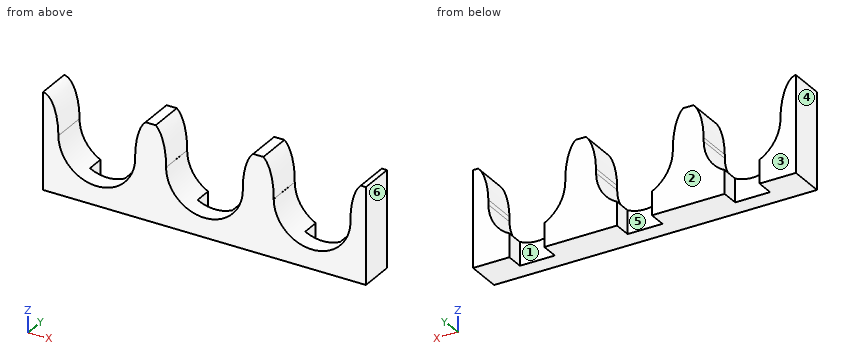
from build123d import *

# Parameters (mm, degrees)
SKETCH1_W           = 469.9
SKETCH1_H           = 139.7
BOSS_EXTRUDE1_DEPTH = 50.8
SKETCH2_R           = 55.88
CUT_EXTRUDE3_DEPTH  = 405.871109401
CUT_EXTRUDE5_DEPTH  = 405.871109401
SKETCH5_W           = 50.8
SKETCH5_H           = 25.4
CUT_EXTRUDE6_DEPTH  = 419.118003235


with BuildPart() as part:
    # Sketch1 → Boss-Extrude1 (new body)
    with BuildSketch(Plane(origin=(0, 0, 0), x_dir=(1, 0, 0), z_dir=(0, 1, 0))):
        with Locations((155.851656231, -22.96185654)):
            Rectangle(SKETCH1_W, SKETCH1_H)
    extrude(amount=BOSS_EXTRUDE1_DEPTH)

    # Sketch2 → Cut-Extrude3 (cut, through all)
    with BuildSketch(Plane(origin=(0, 50.8, 0), x_dir=(1, 0, 0), z_dir=(0, 1, 0))):
        with BuildLine():
            Line((55.098238231, -92.81185654), (55.098238231, -36.93185654))
            ThreePointArc((55.098238231, -36.93185654), (38.731365092, -76.444983544), (-0.781761972, -92.81185654))
            Line((-0.781761972, -92.81185654), (55.098238231, -92.81185654))
        make_face()
        with BuildLine():
            ThreePointArc((-0.781761972, -92.81185654), (-40.294888773, -76.4449834), (-56.661761769, -36.93185654))
            Line((-56.661761769, -36.93185654), (-56.661761769, -92.81185654))
            Line((-56.661761769, -92.81185654), (-0.781761972, -92.81185654))
        make_face()
        with BuildLine():
            Line((99.971656231, -36.93185654), (99.971656231, -92.81185654))
            Line((99.971656231, -92.81185654), (155.851656231, -92.81185654))
            ThreePointArc((155.851656231, -92.81185654), (116.338529299, -76.444983472), (99.971656231, -36.93185654))
        make_face()
        with BuildLine():
            ThreePointArc((211.731656231, -36.93185654), (195.364783164, -76.444983472), (155.851656231, -92.81185654))
            Line((155.851656231, -92.81185654), (211.731656231, -92.81185654))
            Line((211.731656231, -92.81185654), (211.731656231, -36.93185654))
        make_face()
        with BuildLine():
            Line((256.605074231, -36.93185654), (256.605074231, -92.81185654))
            Line((256.605074231, -92.81185654), (312.485074664, -92.81185654))
            ThreePointArc((312.485074664, -92.81185654), (272.971947451, -76.444983625), (256.605074231, -36.93185654))
        make_face()
        with BuildLine():
            ThreePointArc((368.365074231, -36.93185654), (351.998201317, -76.444983319), (312.485074664, -92.81185654))
            Line((312.485074664, -92.81185654), (368.365074231, -92.81185654))
            Line((368.365074231, -92.81185654), (368.365074231, -36.93185654))
        make_face()
        with Locations((312.485074231, -36.93185654)):
            Circle(SKETCH2_R)
        with Locations((155.851656231, -36.93185654)):
            Circle(SKETCH2_R)
        with Locations((-0.781761769, -36.93185654)):
            Circle(SKETCH2_R)
    extrude(amount=-CUT_EXTRUDE3_DEPTH, mode=Mode.SUBTRACT)

    # Sketch3 → Cut-Extrude5 (cut, through all)
    with BuildSketch(Plane(origin=(0, 50.8, 0), x_dir=(1, 0, 0), z_dir=(0, 1, 0))):
        with BuildLine():
            Line((-56.661761769, -92.81185654), (-56.661761769, -36.93185654))
            add(Edge.make_bspline(
                [(-79.098343769, -92.81185654), (-56.661761769, -92.81185654), (-56.661761769, -36.93185654)],
                knots=[0, 0, 0, 1.570796327, 1.570796327, 1.570796327], degree=2, weights=[1, 0.707106781, 1]))
            Line((-79.098343769, -92.81185654), (-56.661761769, -92.81185654))
        make_face()
        with BuildLine():
            add(Edge.make_bspline(
                [(55.098238231, -42.266592873), (55.687318095, -80.198521665), (70.062894281, -92.81185654)],
                knots=[4.75104815, 4.75104815, 4.75104815, 5.944468502, 5.944468502, 5.944468502], degree=2, weights=[1, 0.82718872, 1]))
            Line((55.098238231, -42.266592873), (55.098238231, -92.81185654))
            Line((55.098238231, -92.81185654), (70.062894281, -92.81185654))
        make_face()
        with BuildLine():
            Line((99.971656231, -36.93185654), (99.918392881, -36.93185654))
            add(Edge.make_bspline(
                [(84.973218182, -92.81185654), (100.8764169, -78.858163942), (99.918392881, -36.93185654)],
                knots=[0.338716805, 0.338716805, 0.338716805, 1.627645124, 1.627645124, 1.627645124], degree=2, weights=[1, 0.799421799, 1]))
            Line((84.973218182, -92.81185654), (99.971656231, -92.81185654))
            Line((99.971656231, -92.81185654), (99.971656231, -36.93185654))
        make_face()
        with BuildLine():
            add(Edge.make_bspline(
                [(211.731656231, -43.172150916), (212.553221033, -80.41743909), (226.679294281, -92.81185654)],
                knots=[4.767271474, 4.767271474, 4.767271474, 5.944468502, 5.944468502, 5.944468502], degree=2, weights=[1, 0.831719595, 1]))
            Line((211.731656231, -43.172150916), (211.731656231, -92.81185654))
            Line((211.731656231, -92.81185654), (226.679294281, -92.81185654))
        make_face()
        with BuildLine():
            Line((256.605074231, -36.93185654), (256.534792881, -36.93185654))
            add(Edge.make_bspline(
                [(241.589618182, -92.81185654), (257.4928169, -78.858163942), (256.534792881, -36.93185654)],
                knots=[0.338716805, 0.338716805, 0.338716805, 1.627645124, 1.627645124, 1.627645124], degree=2, weights=[1, 0.799421799, 1]))
            Line((241.589618182, -92.81185654), (256.605074231, -92.81185654))
            Line((256.605074231, -92.81185654), (256.605074231, -36.93185654))
        make_face()
        with BuildLine():
            add(Edge.make_bspline(
                [(368.365074231, -43.865048297), (369.358856755, -80.583477202), (383.295694281, -92.81185654)],
                knots=[4.779694469, 4.779694469, 4.779694469, 5.944468502, 5.944468502, 5.944468502], degree=2, weights=[1, 0.835152126, 1]))
            Line((368.365074231, -43.865048297), (368.365074231, -92.81185654))
            Line((368.365074231, -92.81185654), (383.295694281, -92.81185654))
        make_face()
    extrude(amount=-CUT_EXTRUDE5_DEPTH, mode=Mode.SUBTRACT)

    # Sketch5 → Cut-Extrude6 (cut, through all)
    with BuildSketch(Plane(origin=(0, 0, -46.88814346), x_dir=(-1, 0, 0), z_dir=(0, 0, -1))):
        with Locations((-312.485836231, 38.1)):
            Rectangle(SKETCH5_W, SKETCH5_H)
        with Locations((-155.851656231, 38.1)):
            Rectangle(SKETCH5_W, SKETCH5_H)
        with Locations((0.782523769, 38.1)):
            Rectangle(SKETCH5_W, SKETCH5_H)
    extrude(amount=-CUT_EXTRUDE6_DEPTH, mode=Mode.SUBTRACT)


solid = part.part
Geometry: final body of the model. Coordinates: model frame, mm. Face numbers are marked on the shaded views. A direction names the side the tool comes from. Give positions to 0.01 mm unless a question says otherwise; leave off trailing zeros. Order: outer loops, then holes, each group sorted by start corner. A loop starts at its lowest first (then second) coordinate and runs counter-clockwise, first axis right, second up. Notation, with made-up numbers: (21.25, 66) -> (28.25, 66) arc R26 cw to (28.25, 93) -> close; hole circle Ø2 at (-9, -38.5). An arc over 180 degrees is marked (long way). Answer as a JSON object with one key per item and string values.
Q1. Section A-A (z = -1). Output: boundary loops of the cut face in (x, y).
Entries:
{"outline": "(-79.1, 0) -> (-41.82, 0) -> (-41.82, 50.8) -> (-79.1, 50.8) -> close; (40.25, 0) -> (114.82, 0) -> (114.82, 50.8) -> (40.25, 50.8) -> close; (196.89, 0) -> (271.45, 0) -> (271.45, 50.8) -> (196.89, 50.8) -> close; (353.52, 0) -> (390.8, 0) -> (390.8, 50.8) -> (353.52, 50.8) -> close"}
Q2. Access query for the marked faces 1 and 2. Directions: +Z, -Z, +X, -X, +Y, -Y. A direction counts if a zero-diameter tool reaches every point of the face in a straight line with its end or side. Return the directions, or none.
Entries:
{"face 1": "+Z, -Z, +Y", "face 2": "+Z, -Z, +X, -X, +Y"}
Q3. Material intervals for probe 1 along X at (y, z) = (31, -21.5); probe 2 along X at (y, z) = (10, 41.5); probe 3 along Y at (x, z) = (22.5, -23), sorted ascending.
Entries:
{"probe 1": "x = -79.1 to -26.18, 24.62 to 130.45, 181.25 to 287.09, 337.89 to 390.8", "probe 2": "x = -79.1 to -56.74, 55.1 to 99.95, 211.73 to 256.56, 368.37 to 390.8", "probe 3": "y = 0 to 25.4"}
Q4. Draft query along X for the marked faces 3, 4, 5 and 6. Return one class per face: released by +X, released by -X, zero draft, split by the parting line, or undercut.
Entries:
{"face 3": "zero draft", "face 4": "released by -X", "face 5": "undercut", "face 6": "released by +X"}
Q5. Section B-B (z = -31.5). Output: boundary loops of the cut face in (x, y), plus the area to 3 significant figures.
Entries:
{"outline": "(-79.1, 0) -> (390.8, 0) -> (390.8, 50.8) -> (337.89, 50.8) -> (337.89, 25.4) -> (287.09, 25.4) -> (287.09, 50.8) -> (181.25, 50.8) -> (181.25, 25.4) -> (130.45, 25.4) -> (130.45, 50.8) -> (24.62, 50.8) -> (24.62, 25.4) -> (-26.18, 25.4) -> (-26.18, 50.8) -> (-79.1, 50.8) -> close", "area": "20,000 mm^2"}
Q6. First-contact query: pin 1 (4 mm diameter, centred on x = 60.5, z = -25.5, fed in from -Y); pin 2 (10 mm diameter, centred on x = 167, z = -25, fed in from +Y). Flat tips, straight axial feed; report the tip coordinate or a pass-through.
Entries:
{"pin 1": "stops at y = 0", "pin 2": "stops at y = 25.4"}
Q7. Section C-C (z = 25.5). Output: boundary loops of the cut face in (x, y), plus the area to 3 significant figures.
Entries:
{"outline": "(-79.1, 0) -> (-55.48, 0) -> (-55.48, 50.8) -> (-79.1, 50.8) -> close; (53.92, 0) -> (101.15, 0) -> (101.15, 50.8) -> (53.92, 50.8) -> close; (210.55, 0) -> (257.79, 0) -> (257.79, 50.8) -> (210.55, 50.8) -> close; (367.18, 0) -> (390.8, 0) -> (390.8, 50.8) -> (367.18, 50.8) -> close", "area": "7,200 mm^2"}
Q8. Section D-D (x = 122.5). Output: boundary loops of the cut face in (y, z).
Entries:
{"outline": "(0, -46.89) -> (50.8, -46.89) -> (50.8, -7.9) -> (0, -7.9) -> close"}
